```python
from build123d import *

# Parameters (mm, degrees)
SKETCH1_OUTSIDE_W   = 3521.15
SKETCH1_OUTSIDE_H   = 3521.15
SKETCH1_OUTSIDE_W_2 = 203.2
SKETCH1_OUTSIDE_H_2 = 203.2
CUT_EXTRUDE1_DEPTH  = 2190.743594482
CUT_EXTRUDE2_START  = 3.175
SKETCH5_W           = 234.523944536
SKETCH5_H           = 253.300586876
CUT_EXTRUDE2_DEPTH  = 1052.463791587
SKETCH6_R           = 3.4925
SKETCH6_W           = 127
SKETCH6_H           = 127
CUT_EXTRUDE3_DEPTH  = 144.719172925


with BuildPart() as part:
    # Sketch3 → Revolve1 (revolve)
    with BuildSketch(Plane(origin=(0, 0, 0), x_dir=(0, 0, -1), z_dir=(1, 0, 0))):
        with BuildLine():
            Line((0, 0), (0, 1044.805178237))
            add(Edge.make_bspline(
                [(0, 1044.805178237), (-1360.764334547, 1044.805178237), (-1360.764334547, 522.402589118), (-1360.764334547, 0), (0, 0)],
                knots=[1.570796327, 1.570796327, 1.570796327, 3.141592654, 3.141592654, 4.71238898, 4.71238898, 4.71238898], degree=2, weights=[1, 0.707106781, 1, 0.707106781, 1]))
        make_face()
    revolve(axis=Axis((0, 0, 0), (0, 1, 0)))

    # Sketch1 outside → Cut-Extrude1 (cut, through all)
    with BuildSketch(Plane(origin=(0, 0, 0), x_dir=(1, 0, 0), z_dir=(0, 1, 0))):
        Rectangle(SKETCH1_OUTSIDE_W, SKETCH1_OUTSIDE_H)
        Rectangle(SKETCH1_OUTSIDE_W_2, SKETCH1_OUTSIDE_H_2, mode=Mode.SUBTRACT)
    extrude(amount=CUT_EXTRUDE1_DEPTH, mode=Mode.SUBTRACT)

    # Sketch5 → Cut-Extrude2 (cut, through all)
    with BuildSketch(Plane(origin=(0, 0, 0), x_dir=(1, 0, 0), z_dir=(0, 1, 0)).offset(CUT_EXTRUDE2_START)):
        Rectangle(SKETCH5_W, SKETCH5_H)
    extrude(amount=CUT_EXTRUDE2_DEPTH, mode=Mode.SUBTRACT)

    # Sketch6 → Cut-Extrude3 (cut, through all)
    with BuildSketch(Plane(origin=(0, 3.175, 0), x_dir=(1, 0, 0), z_dir=(0, 1, 0))):
        with Locations(Location((-95.25, -95.25, 0), (0, 0, 270))):
            Circle(SKETCH6_R)
        with Locations(Location((-95.25, 95.25, 0), (0, 0, 270))):
            Circle(SKETCH6_R)
        with Locations(Location((95.25, 95.25, 0), (0, 0, 270))):
            Circle(SKETCH6_R)
        with Locations(Location((95.25, -95.25, 0), (0, 0, 270))):
            Circle(SKETCH6_R)
        Rectangle(SKETCH6_W, SKETCH6_H)
    extrude(amount=-CUT_EXTRUDE3_DEPTH, mode=Mode.SUBTRACT)


solid = part.part
```
Here's how the part is built. I have some questions about the finished solid (model axes, mm). Round coordinates to 2 decimals unless told otherwise and drop trailing zeros.
1. Thinking about a two-plate mould opening in Z: for faces 1 (the face through (-94.2, 2.89, -91.92)), 2 (the face through (-1, 3.175, 66)), which applies, released by +Z, released by -Z, zero draft, split by the parting line, or undercut?
Answers:
face 1: undercut
face 2: zero draft
2. If I drill on probe 1 along X at (y, z) = (2.9, 95.25); probe 2 along Z at (x, y) = (-32, 2.9), over which ranges is the centre line in solid material (lowest first)?
Answers:
probe 1: x = -101.6 to -98.74, -91.76 to 91.76, 98.74 to 101.6
probe 2: z = -101.6 to -63.5, 63.5 to 101.6
3. Will these pins go through, and if not, where does the flat tip stop? pin 1 (11 mm diameter, centred on x = -95.25, z = -95.25, fed in from -Y); pin 2 (4 mm diameter, centred on x = 95.25, z = -95.25, fed in from -Y).
Answers:
pin 1: stops at y = 2.36
pin 2: passes through
4. Suppose I cut it at A-A, the plane z = -95.25. Give the number of separate pieces and of enclosed holes in the cut face, and give its area (3 significant figures).
Answers:
separate pieces: 3
enclosed holes: 0
area: 277 mm2
